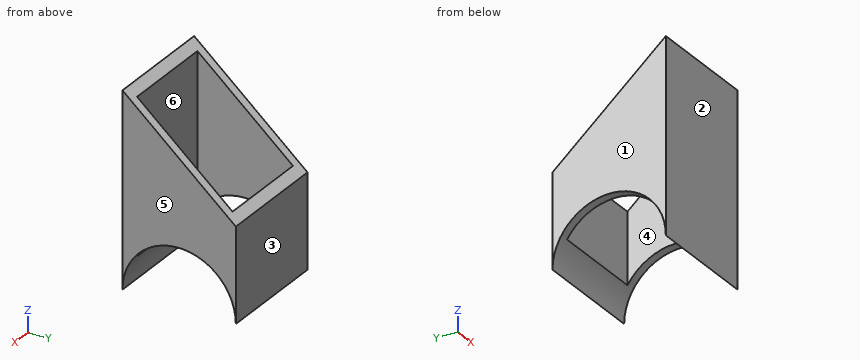
from build123d import *

# Parameters (mm, degrees)
F1_DEPTH = 12.7
F2_T     = -2
F4_DEPTH = 29.083


with BuildPart() as f1:
    # F0 (on Right) → F1 (new body, symmetric)
    with BuildSketch(Plane.YZ):
        Polygon((-12.7, 21.5), (-12.7, -21.5), (12.7, -21.5), (12.7, -0.5), align=None)
    extrude(amount=F1_DEPTH, both=True)

    # F2
    f2_openings = [f1.faces().sort_by_distance(p)[0] for p in [
        (0, 0, -21.5),
        (0, 0, 10.5),
    ]]
    offset(amount=F2_T, openings=f2_openings)

    # F3 (on face) → F4 (cut)
    with BuildSketch(Plane.YZ.offset(12.7)):
        with BuildLine():
            Line((-12.7, -21.5), (12.7, -21.5))
            ThreePointArc((12.7, -21.5), (0, -8.8), (-12.7, -21.5))
        make_face()
    extrude(amount=-F4_DEPTH, mode=Mode.SUBTRACT)


solid = f1.part
Design review of the part built by this model. Coordinates are the model's own, in mm. Face numbers are marked on the shaded views. A direction names the side the tool comes from. Coordinates: 2 decimals unless noted, no trailing zeros. Order: outer loops, then holes, each group sorted by start corner. A loop starts at its lowest first (then second) coordinate and runs counter-clockwise, first axis right, second up.
Item 1: Take a section at C-C, the plane z = 16. Write out the cut boundary in (x, y), then the cut area to 3 significant figures.
Item 2: Take a section at A-A, the plane x = -10. Write out the cut boundary in (y, z), then the cut area to 3 significant figures.
Item 3: The part is to be moulded in two halves that separate along Y. For the marked faces 1, 2, 3 and 4, say which applies: pulls with the +Y half, pulls with the -Y half, needs draft (parallel to the pull), parting line crosses it, or undercut.
Item 4: For line 1 (X direction, y = -7, z = -0.5); line 2 (Y direction, x = 4.5, z = 10), list the stretches that pass through material, from the lowest coordinate up.
Item 5: Take a section at B-B, the plane y = 0. Write out the cut boundary in (x, z), then the cut area to 3 significant figures.
Item 6: For the marked faces 5 and 6, list the 3-axis set-ups (+Z, -Z, +X, -X, +Y, -Y) from which the entire face can be reached by the end or side of a thin tool; tool diameter is ignored.
The answers:
1. outline: (-12.7, -12.7) - (12.7, -12.7) - (12.7, -6.35) - (10.7, -6.35) - (10.7, -10.7) - (-10.7, -10.7) - (-10.7, -6.35) - (-12.7, -6.35) - close
1. area: 68.2 mm2
2. outline: (-12.7, -21.5) arc R12.7 cw to (-10.7, -14.66) - (-10.7, 19.77) - (-12.7, 21.5) - close; (10.7, -14.66) arc R12.7 cw to (12.7, -21.5) - (12.7, -0.5) - (10.7, 1.23) - close
2. area: 109 mm2
3. face 1: needs draft
3. face 2: pulls with the -Y half
3. face 3: pulls with the +Y half
3. face 4: undercut
4. line 1: x = -12.7 to -10.7, 10.7 to 12.7
4. line 2: y = -12.7 to -10.7
5. outline: (-12.7, -8.8) - (-10.7, -8.8) - (-10.7, 10.5) - (-12.7, 10.5) - close; (10.7, -8.8) - (12.7, -8.8) - (12.7, 10.5) - (10.7, 10.5) - close
5. area: 77.2 mm2
6. face 5: +Z, -Z, +X, +Y, -Y
6. face 6: +Z, -Z
